Study the drawing (mm; zero at the part's minimum x, y, z) and answer. A direction names the side the tool comes from. Round coordinates to 2 decimals unless told otherwise and drop trailing zeros. Order: outer loops, then holes, each group sorted by start corner. A loop starts at its lowest first (then second) coordinate and runs counter-clockwise, first axis right, second up. Notation, with made-up numbers: (6, 51) - (39, 51) arc R35 cw to (39, 84) - close; hole circle Ø5 at (88.25, 46.5). An arc over 180 degrees is marked (long way). Use one line per item in the form item = value. Start each with the question number.
Q1. For a pull along X with two mould halves and no side action, classify the marked faces 5, 6 and 7 as +X half, -X half, draft (parallel to the pull), parting line (faces both ways), or undercut.
Q2. The part is cut by section A-A on y = 56. Determine the outline of the cut face in (x, z) (3 decimals), plus the area to 3 significant figures.
Q3. Given P1, Ø8, axis at y = 9.525, z = 15.24, coming from the +X side; P2, Ø9.5, axis at x = 15.5, y = 78.5, coming from the +Z side (3 decimals); P3, Ø10, axis at x = 89.5, z = 16, coming from the -Y side, each flat-ended and moving along its own axis, determine where each tip first touches the part or whether it passes through.
Q4. The part is cut by section B-B on x = 28. Determine the outline of the cut face in (y, z), plus the area to 3 significant figures.
Q5. Find the intervals of material crossed by line 1 (X direction, y = 24, z = 22.5); line 2 (Y direction, x = 138, z = 15); line 3 (Y direction, x = 93.5, z = 9), in increasing order. Write a range as [from, to].
Q6. Which of the six approach directions +Z, -Z, +X, -X, +Y, -Y give full straight-line access (tool end or side, diameter ignored) to the marked faces 1, 2, 3 and 4?
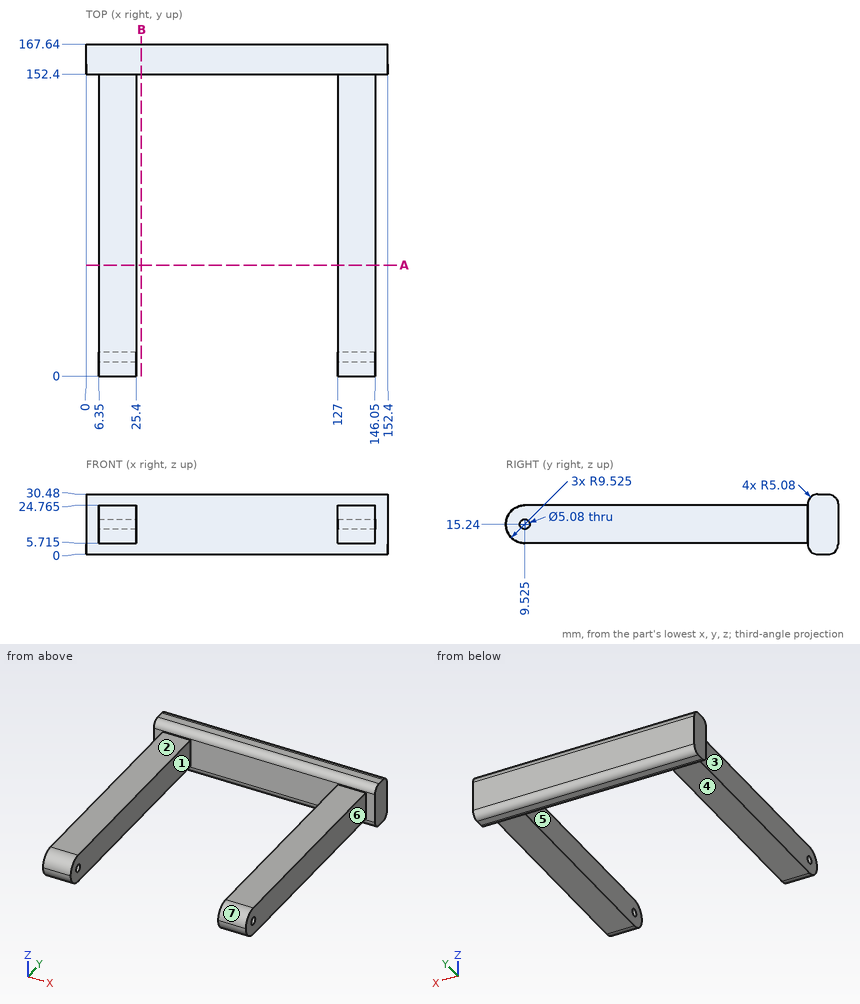
Found:
q1.face_5 = undercut
q1.face_6 = +X half
q1.face_7 = draft
q2.outline = (6.35, 5.715) - (25.4, 5.715) - (25.4, 24.765) - (6.35, 24.765) - close; (127, 5.715) - (146.05, 5.715) - (146.05, 24.765) - (127, 24.765) - close
q2.area = 726 mm²
q3.P1 = 146.05
q3.P2 = 24.765
q3.P3 = 152.4
q4.outline = (152.4, 5.08) arc R5.08 ccw to (157.48, 0) - (162.56, 0) arc R5.08 ccw to (167.64, 5.08) - (167.64, 25.4) arc R5.08 ccw to (162.56, 30.48) - (157.48, 30.48) arc R5.08 ccw to (152.4, 25.4) - close
q4.area = 442 mm²
q5.line_1 = [6.35, 25.4], [127, 146.05]
q5.line_2 = [0, 7], [12.05, 167.64]
q5.line_3 = [152.4, 167.64]
q6.face_1 = +Z, -Z, -Y
q6.face_2 = +Z, +X, -X, -Y
q6.face_3 = +Z, -Z, -X, -Y
q6.face_4 = -Z, +X, -X, -Y
